Source: CAD feature listing. Evaluate the final solid. Frame: model axes, mm. A direction names the side the tool comes from. Give positions to 0.01 mm unless a question says otherwise; leave off trailing zeros. Order: outer loops, then holes, each group sorted by start corner. A loop starts at its lowest first (then second) coordinate and runs counter-clockwise, first axis right, second up. Notation, with made-up numbers: (42.25, 73) - (97.25, 73) arc R16 ccw to (97.25, 97) - close; hole circle Ø6 at (-8, 88). An arc over 180 degrees is marked (long way). Write each question's results on one line, items separated by ' | '. Start each with the question number.
Item 1: Section A-A on y = 53. Output: boundary loops of the cut face in (x, z), and give its area (3 significant figures).
Item 2: Set-up query: faces 1 (the cylindrical face through (-0.176, 67.998, -0.493)), 2 (the flat face through (16, 30, 0)), 3 (the flat face through (-48.095, 29.58, 60.84)), 4 (the flat face through (49, 0, 60)), 5 (the flat face through (-17, 30, 0)). Return all of +Z, -Z, +X, -X, +Y, -Y with unobstructed straight access to the full face (end or side cutting, diameter ignored); none if empty.
Item 3: Section B-B on z = 18. Output: boundary loops of the cut face in (x, y), and give its area (3 significant figures).
Item 4: Line query: line 1 along Z through (x, y) = (-21, 18.5); line 2 along X through (y, z) = (87.5, 78); line 3 along X through (y, z) = (41, 76.5). Output: solid intervals per line, ascending.
Item 5: Section D-D on z = 73. Output: boundary loops of the cut face in (x, y).
Item 6: Contact query for flat-ended pins moving along their axis: pin 1 Ø1 at (y, z) = (60, 87) entering from -X; pin 2 Ø0.8 at (y, z) = (23, -0.5) entering from +X; pin 3 Ø6 at (x, z) = (-3.5, 93) entering from +Y. Output: stop coordinate, or through.
Item 7: Mould query, pull axis Z, two halves, no side actions, for faces 6 (the flat face through (-49, 0, 60)), 7 (the conical face through (0.916, 101.64, 47.507)), 8 (the flat face through (51.095, 29.58, 60.84)). Classes: released by +Z, released by -Z, zero draft, split by the parting line, or undercut.
```python
from build123d import *

# Parameters (mm, degrees)
F4_W     = 17
F4_H     = 60
F4_W_2   = 3
F5_DEPTH = 1


with BuildPart() as f3:
    # F0 (on Top) → F3 section 0
    with BuildSketch(Plane.XY):
        with BuildLine():
            Line((5, 60), (5, 0))
            Line((5, 0), (8, 0))
            Line((8, 0), (8, 60))
            ThreePointArc((8, 60), (0, 68), (-8, 60))
            Line((-8, 60), (-8, 0))
            Line((-8, 0), (-5, 0))
            Line((-5, 0), (-5, 60))
            ThreePointArc((-5, 60), (0, 65), (5, 60))
        make_face()
    # F2 (on offset) → F3 section 1
    with BuildSketch(Plane.XY.offset(120)):
        with BuildLine():
            Line((-90, 0), (-90, 60))
            ThreePointArc((-90, 60), (0, 150), (90, 60))
            Line((90, 60), (90, 0))
            Line((90, 0), (93, 0))
            Line((93, 0), (93, 60))
            ThreePointArc((93, 60), (0, 153), (-93, 60))
            Line((-93, 60), (-93, 0))
            Line((-93, 0), (-90, 0))
        make_face()
    loft()

    # F4 (on face) → F5 (join)
    with BuildSketch(Plane(origin=(0, 0, 0), x_dir=(1, 0, 0), z_dir=(0, 0, -1))):
        with BuildLine():
            ThreePointArc((5, -60), (0, -65), (-5, -60))
            Line((-5, -60), (-8, -60))
            ThreePointArc((-8, -60), (0, -68), (8, -60))
            Line((8, -60), (5, -60))
        make_face()
        with Locations((-16.5, -30)):
            Rectangle(F4_W, F4_H)
        with Locations((16.5, -30)):
            Rectangle(F4_W, F4_H)
        with Locations((6.5, -30)):
            Rectangle(F4_W_2, F4_H)
        with Locations((-6.5, -30)):
            Rectangle(F4_W_2, F4_H)
    extrude(amount=F5_DEPTH)


solid = f3.part
```
Evaluation:
1) outline: (-93, 120) - (-8, 0) - (-25, 0) - (-25, -1) - (-5, -1) - (-5, 0) - (-90, 120) - close; (5, -1) - (25, -1) - (25, 0) - (8, 0) - (93, 120) - (90, 120) - (5, 0) - close | area: 760 mm^2
2) face 1: -Z, +Y | face 2: +X, +Y, -Y | face 3: +Z, -Y | face 4: +Z, -Z, +X, -X, -Y | face 5: -X, +Y, -Y
3) outline: (-20.75, 0) - (-17.75, 0) - (-17.75, 60) arc R17.75 cw to (17.75, 60) - (17.75, 0) - (20.75, 0) - (20.75, 60) arc R20.75 ccw to (-20.75, 60) - close | area: 541 mm^2
4) line 1: z = -1 to 0, 18.35 to 22.59 | line 2: x = -56.96 to -53.61, 53.61 to 56.96 | line 3: x = -62.19 to -59.19, 59.19 to 62.19
5) outline: (-59.71, 0) - (-56.71, 0) - (-56.71, 60) arc R56.71 cw to (56.71, 60) - (56.71, 0) - (59.71, 0) - (59.71, 60) arc R59.71 ccw to (-59.71, 60) - close
6) pin 1: stops at x = -69.98 | pin 2: stops at x = 25 | pin 3: stops at y = 135.92
7) face 6: zero draft | face 7: released by -Z | face 8: undercut
